Geometry check sheet. Reference: drawing and pictorial views, mm from the part's lowest x, y, z. Coordinates: 2 decimals unless noted, no trailing zeros. Loops run counter-clockwise (first coordinate to the right, second up) from the corner with the lowest first, then second, coordinate; pieces in that order, holes last. Notation, with made-up numbers: M 6.25,79.25 L 26.25,79.25 A24 cw 26.25,93.25 Z; hole C 56,25.5 d3. An arc over 180 degrees is marked long. Write each question's results on one line, items separated by ' | '. Start each with the question number.
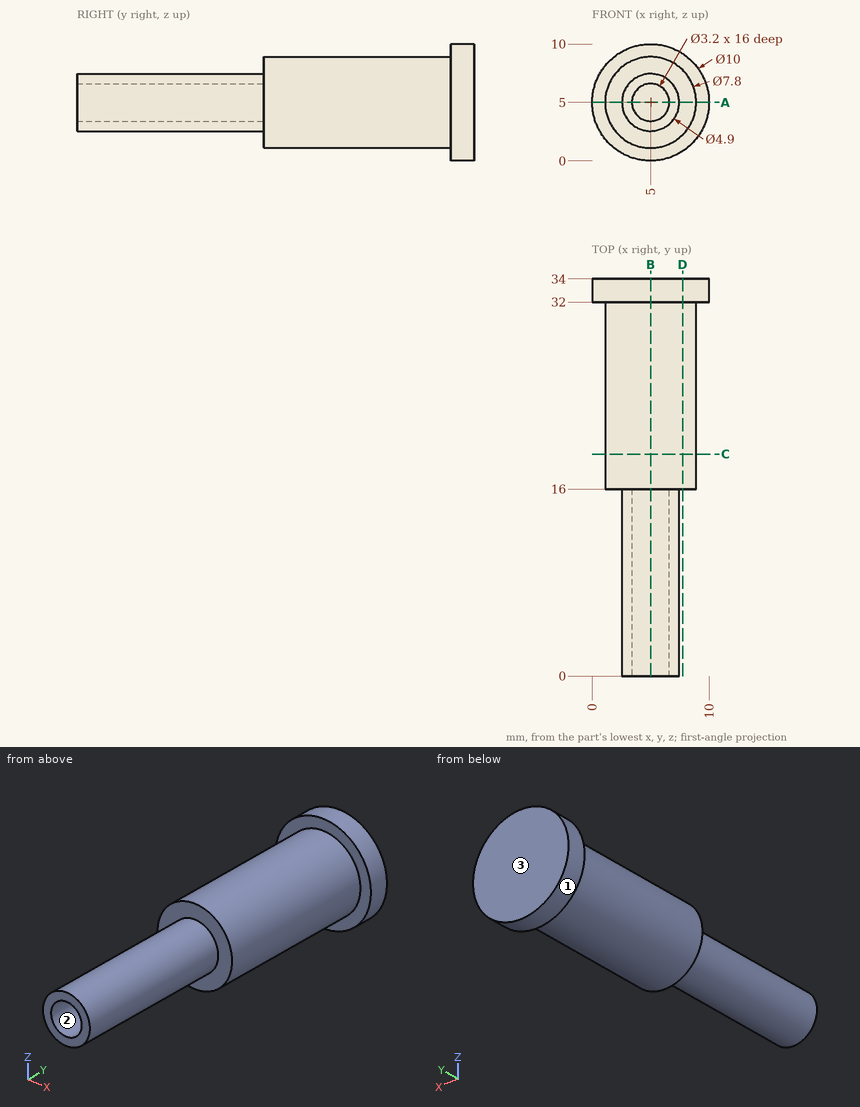
1) Section check C-C (y = 19). Enter the section's corners in (x, z).
2) Gauge pin test, flat ends, axial feed: P1, Ø4, axis at y = 5, z = 4.5, coming from the -X side; P2, Ø4, axis at x = 7.5, y = 21, coming from the +Z side; P3, Ø4, axis at x = 6, z = 6, coming from the -Y side; P4, Ø1, axis at x = 4.5, z = 5, coming from the -Y side. Record the tip position at first contact, or that the pin passes through.
3) Section check B-B (x = 5). Enter the section's corners in (y, z).
4) Section check D-D (x = 7.75). Enter the section's corners in (y, z), then the cut area to 3 significant figures.
5) Thickness scan on probe 1 along X at (y, z) = (12.5, 5); probe 2 along Y at (x, z) = (7.75, 3). Record the ranges inside material, lowest first.
6) Release check for a two-part mould opening along Z. For the marked faces 1, 2 and 3 record: +Z half, -Z half, draft (parallel to the pull), parting line (faces both ways), or undercut.
7) Section check A-A (z = 5). Enter the section's corners in (x, y).
Return value:
1) outline: C 5,5 d7.8
2) P1: stops at x = 2.55 | P2: stops at z = 8.87 | P3: stops at y = 0 | P4: stops at y = 16
3) outline: M 0,2.55 L 16,2.55 L 16,1.1 L 32,1.1 L 32,0 L 34,0 L 34,10 L 32,10 L 32,8.9 L 16,8.9 L 16,7.45 L 0,7.45 L 0,6.6 L 16,6.6 L 16,3.4 L 0,3.4 Z
4) outline: M 16,2.23 L 32,2.23 L 32,0.82 L 34,0.82 L 34,9.18 L 32,9.18 L 32,7.77 L 16,7.77 Z | area: 105 mm2
5) probe 1: x = 2.55 to 3.4, 6.6 to 7.45 | probe 2: y = 16 to 34
6) face 1: parting line | face 2: undercut | face 3: draft
7) outline: M 0,32 L 1.1,32 L 1.1,16 L 2.55,16 L 2.55,0 L 3.4,0 L 3.4,16 L 6.6,16 L 6.6,0 L 7.45,0 L 7.45,16 L 8.9,16 L 8.9,32 L 10,32 L 10,34 L 0,34 Z
